Part model, mm, in its own coordinate system. Face numbers are marked on the shaded views. A direction names the side the tool comes from. Round coordinates to 2 decimals unless told otherwise and drop trailing zeros. Loops run counter-clockwise (first coordinate to the right, second up) from the corner with the lowest first, then second, coordinate; pieces in that order, holes last.
1) Band-saw the part on B-B, the plane x = 19. Write the cut outline in (y, z) (3 decimals).
2) Band-saw the part on D-D, the plane x = 9. State how many separate pieces and enclosed holes the cut face has, then the cut area to 3 significant figures.
3) Drop flat-ended pins along their axis: P1, Ø11, axis at x = 9.525, z = -34.925, coming from the +Y side; P2, Ø5, axis at x = 16.5, z = -22.5, coming from the +Y side (3 decimals); P3, Ø2, axis at y = 43, z = -59.5, coming from the -X side. Give the stop position or say it passes through.
4) Band-saw the part on A-A, the plane z = -58.5. Write the cut outline in (x, y) (1 decimal), then the cut area to 3 significant figures.
5) 3-axis set-ups, long thin cutter, end or side, ignore diameter. For the marked faces 1 and 2: which of +Z, -Z, +X, -X, +Y, -Y reach the whole face in a straight line?
6) Probe line 1 (X direction, y = 100.5, z = -28); line 2 (Y direction, x = 15.5, z = -55.5) (3 decimals); line 3 (Y direction, x = 30.5, z = -50.5). List the from-to ranges inside material, lowest first.
7) Band-saw the part on C-C, the plane y = 17.5. Write the cut outline in (x, z).
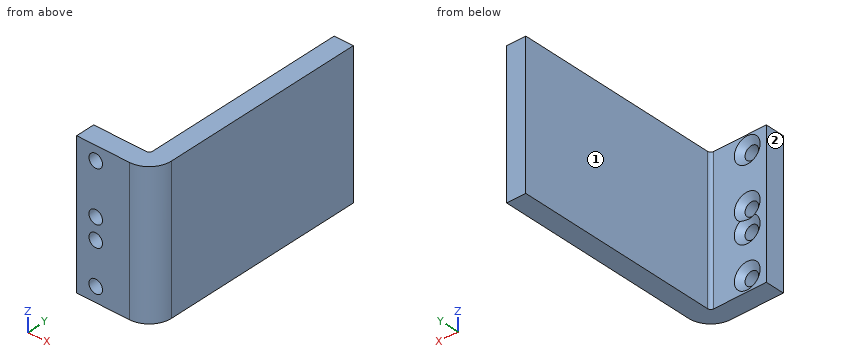
from build123d import *

# Parameters (mm, degrees)
SKETCH1_W                                           = 25.4
SKETCH1_H                                           = 71.12
BOSS_EXTRUDE1_DEPTH                                 = 9.525
CSK_FOR_1_4_FLAT_HEAD_MACHINE_SCREW_100_D           = 6.7564
CSK_FOR_1_4_FLAT_HEAD_MACHINE_SCREW_100_CSINK_D     = 12.8778
CSK_FOR_1_4_FLAT_HEAD_MACHINE_SCREW_100_CSINK_ANGLE = 100
SKETCH6_W                                           = 71.12
SKETCH6_H                                           = 9.525


with BuildPart() as part:
    # Sketch1 → Boss-Extrude1 (new body)
    with BuildSketch(Plane(origin=(0, 0, 0), x_dir=(1, 0, 0), z_dir=(0, 1, 0))):
        with Locations((12.7, 38.1)):
            Rectangle(SKETCH1_W, SKETCH1_H)
    extrude(amount=BOSS_EXTRUDE1_DEPTH)

    # CSK for 1/4 Flat Head Machine Screw (100)1 (through all)
    with Locations(Plane(origin=(0, 9.525, 0), x_dir=(1, 0, 0), z_dir=(0, 1, 0))):
        with Locations((9.525, 9.525), (9.525, 34.925), (9.525, 45.4406), (9.525, 66.3194)):
            CounterSinkHole(CSK_FOR_1_4_FLAT_HEAD_MACHINE_SCREW_100_D / 2, CSK_FOR_1_4_FLAT_HEAD_MACHINE_SCREW_100_CSINK_D / 2, counter_sink_angle=CSK_FOR_1_4_FLAT_HEAD_MACHINE_SCREW_100_CSINK_ANGLE)

    # Sweep1: sweep along a path in Sketch4
    with BuildLine(Plane(origin=(0, 0, -73.66), x_dir=(-1, 0, 0), z_dir=(0, 0, -1))) as sweep1_path:
        Line((-32.643415346, 112.7125), (-32.643415346, 11.1125))
        ThreePointArc((-32.643415346, 11.1125), (-30.783543406, 6.622371939), (-26.293415346, 4.7625))
        Line((-26.293415346, 4.7625), (-25.4, 4.7625))
    # Sketch6 → Sweep1 (sweep)
    with BuildSketch(Plane(origin=(25.4, 0, 0), x_dir=(0, 0, -1), z_dir=(1, 0, 0))):
        with Locations((38.1, 4.7625)):
            Rectangle(SKETCH6_W, SKETCH6_H)
    sweep(path=sweep1_path.line)


solid = part.part
Reported:
1. outline: (0, -73.66) - (9.525, -73.66) - (9.525, -2.54) - (0, -2.54) - close
2. separate pieces: 5
2. enclosed holes: 0
2. area: 393 mm2
3. P1: stops at y = 8.74
3. P2: stops at y = 9.525
3. P3: stops at x = 27.88
4. outline: (0, 0) - (26.3, 0) arc R11.1 ccw to (37.4, 11.1) - (37.4, 112.7) - (27.9, 112.7) - (27.9, 11.1) arc R1.6 cw to (26.3, 9.5) - (0, 9.5) - close
4. area: 1,310 mm2
5. face 1: +Z, -Z, -X, +Y
5. face 2: +Z, -Z, -X, +Y, -Y
6. line 1: x = 27.88 to 37.41
6. line 2: y = 0 to 9.525
6. line 3: y = 0.83 to 112.71
7. outline: (27.88, -73.66) - (37.41, -73.66) - (37.41, -2.54) - (27.88, -2.54) - close
